Here's how the part is built. I have some questions about the finished solid (model axes, mm). Give positions to 0.01 mm unless a question says otherwise; leave off trailing zeros. Loops run counter-clockwise (first coordinate to the right, second up) from the corner with the lowest first, then second, coordinate; pieces in that order, holes last. Notation, with made-up numbers: M -7.5,86.5 L 47.5,86.5 A21 ccw 47.5,120.5 Z; hole C 50,-26.75 d3. An arc over 180 degrees is marked long. Write item = value, one per line. Start each with the question number.
```python
from build123d import *

# Parameters (mm, degrees)
SKETCH1_R             = 92.5
BOSS_EXTRUDE1_DEPTH   = 12
SKETCH2_R             = 7.5
CUT_EXTRUDE1_DEPTH    = 132.363998112
SKETCH3_R             = 9.388365159
CUT_EXTRUDE2_DEPTH    = 9.127201
CIRPATTERN1_START     = 2.872799182
CIRPATTERN1_OUTLINE_R = 9.388365159
CIRPATTERN1_DEPTH     = 9.127200818


# Read off the part's stored shape, not the designer's step: CirPattern1
with BuildPart() as part:
    # Sketch1 → Boss-Extrude1 (new body)
    with BuildSketch(Plane(origin=(0, 0, 0), x_dir=(1, 0, 0), z_dir=(0, 1, 0))):
        with Locations(Location((0, 0, 0), (0, 0, 270))):
            Circle(SKETCH1_R)
    extrude(amount=BOSS_EXTRUDE1_DEPTH)

    # Sketch2 → Cut-Extrude1 (cut, through all)
    with BuildSketch(Plane(origin=(0, 0, 0), x_dir=(1, 0, 0), z_dir=(0, 1, 0))):
        with Locations(Location((0, 0, 0), (0, 0, 270))):
            Circle(SKETCH2_R)
    extrude(amount=CUT_EXTRUDE1_DEPTH, mode=Mode.SUBTRACT)

    # Sketch3 → Cut-Extrude2 (cut)
    with BuildSketch(Plane(origin=(0, 12, 0), x_dir=(1, 0, 0), z_dir=(0, 1, 0))):
        with Locations(Location((-39.819354828, 0, 0), (0, 0, 270))):
            Circle(SKETCH3_R)
    extrude(amount=-CUT_EXTRUDE2_DEPTH, mode=Mode.SUBTRACT)

    # CirPattern1 outline → CirPattern1 (cut)
    with BuildSketch(Plane(origin=(0, 0, 0), x_dir=(1, 0, 0), z_dir=(0, 1, 0)).offset(CIRPATTERN1_START)):
        with Locations((0, 39.819354828)):
            Circle(CIRPATTERN1_OUTLINE_R)
        with Locations((39.819354828, 0)):
            Circle(CIRPATTERN1_OUTLINE_R)
        with Locations((0, -39.819354828)):
            Circle(CIRPATTERN1_OUTLINE_R)
    extrude(amount=CIRPATTERN1_DEPTH, mode=Mode.SUBTRACT)


solid = part.part
```
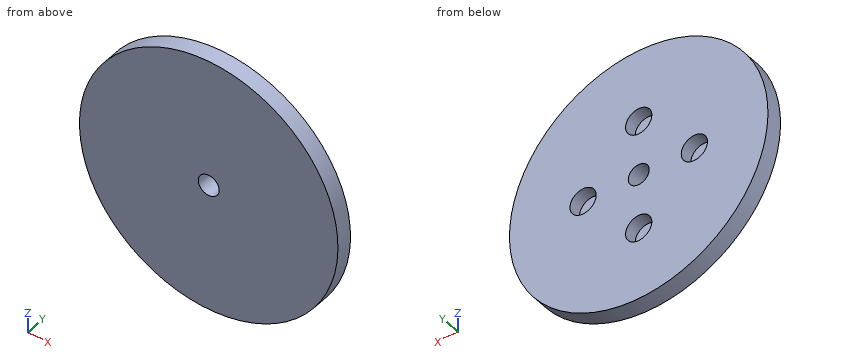
Q1. Will these pins go through, and if not, where does the flat tip stop? pin 1 (2 mm diameter, centred on x = -20.5, y = 2.5, fed in from +Z); pin 2 (2 mm diameter, centred on y = 5.5, z = 48.5, fed in from -X); pin 3 (9.5 mm diameter, centred on x = 0.5, z = -38.5, fed in from +Y).
Q2. If we section it at A-A, the plane z = 0: List the corners of the cut face in (x, y) for me, then the cut area to 3 significant figures.
Q3. If we section it at C-C, the plane y = 10: List the corners of the cut face in (x, z) for me.
Q4. If we section it at D-D, the plane x = 36.5: List the corners of the cut face in (y, z) for me, then the cut area to 3 significant figures.
Q5. If we section it at B-B, the plane x = 0: List the corners of the cut face in (y, z) for me, then the cut area to 3 significant figures.
Q6. If I drill on line 1 along X through (y, z) = (5.25, 0); line 2 along X through (y, z) = (10.5, 1.5); line 3 along Z through (x, y) = (-48, 4.75), over which ranges is the centre line in solid material (lowest first)?
Resolved:
q1.pin_1 = 90.42
q1.pin_2 = -79.37
q1.pin_3 = 2.87
q2.outline = M -92.5,0 L -7.5,0 L -7.5,12 L -30.43,12 L -30.43,2.87 L -49.21,2.87 L -49.21,12 L -92.5,12 Z; M 7.5,0 L 92.5,0 L 92.5,12 L 49.21,12 L 49.21,2.87 L 30.43,2.87 L 30.43,12 L 7.5,12 Z
q2.area = 1,700 mm²
q3.outline = C 0,0 d185; hole C -39.82,0 d18.78; hole C 0,-39.82 d18.78; hole C 0,39.82 d18.78; hole C 0,0 d15; hole C 39.82,0 d18.78
q4.outline = M 0,-84.99 L 12,-84.99 L 12,-8.78 L 2.87,-8.78 L 2.87,8.78 L 12,8.78 L 12,84.99 L 0,84.99 Z
q4.area = 1,880 mm²
q5.outline = M 0,-92.5 L 12,-92.5 L 12,-49.21 L 2.87,-49.21 L 2.87,-30.43 L 12,-30.43 L 12,-7.5 L 0,-7.5 Z; M 0,7.5 L 12,7.5 L 12,30.43 L 2.87,30.43 L 2.87,49.21 L 12,49.21 L 12,92.5 L 0,92.5 Z
q5.area = 1,700 mm²
q6.line_1 = -92.5 to -49.21, -30.43 to -7.5, 7.5 to 30.43, 49.21 to 92.5
q6.line_2 = -92.49 to -49.09, -30.55 to -7.35, 7.35 to 30.55, 49.09 to 92.49
q6.line_3 = -79.07 to -4.61, 4.61 to 79.07
